Model file for the job. Use its own axes, mm. Face numbers are marked on the shaded views. A direction names the side the tool comes from. Coordinates: 2 decimals unless noted, no trailing zeros. Loops run counter-clockwise (first coordinate to the right, second up) from the corner with the lowest first, then second, coordinate; pieces in that order, holes last. Notation, with made-up numbers: (60, 71.25) -> (113, 71.25) arc R8 cw to (113, 78.25) -> close; hole circle Ø4 at (-20.75, 6). An arc over 180 degrees is marked (long way). Use one line per item in the form item = value.
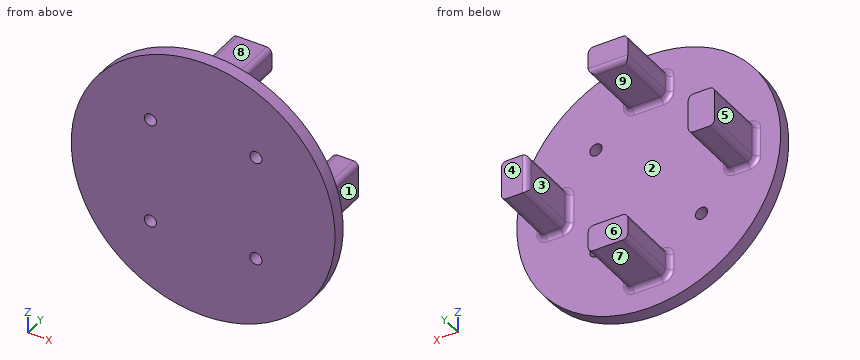
```python
from build123d import *

# Parameters (mm, degrees)
SKETCH2_R           = 63.5
SKETCH2_R_2         = 2.921
BOSS_EXTRUDE2_DEPTH = 6.35
SKETCH3_W           = 19.05
SKETCH3_H           = 12.7
SKETCH3_W_2         = 12.7
SKETCH3_H_2         = 19.05
BOSS_EXTRUDE3_DEPTH = 31.75
FILLET1_R           = 2.54


with BuildPart() as part:
    # Sketch2 → Boss-Extrude2 (new body)
    with BuildSketch(Plane(origin=(0, 0, 0), x_dir=(1, 0, 0), z_dir=(0, 1, 0))):
        with Locations(Location((0, 0, 0), (0, 0, 270))):
            Circle(SKETCH2_R)
        with Locations(Location((-25.4, 25.4, 0), (0, 0, 270))):
            Circle(SKETCH2_R_2, mode=Mode.SUBTRACT)
        with Locations(Location((25.4, 25.4, 0), (0, 0, 270))):
            Circle(SKETCH2_R_2, mode=Mode.SUBTRACT)
        with Locations(Location((25.4, -25.4, 0), (0, 0, 270))):
            Circle(SKETCH2_R_2, mode=Mode.SUBTRACT)
        with Locations(Location((-25.4, -25.4, 0), (0, 0, 270))):
            Circle(SKETCH2_R_2, mode=Mode.SUBTRACT)
    extrude(amount=BOSS_EXTRUDE2_DEPTH)

    # Sketch3 → Boss-Extrude3 (add)
    with BuildSketch(Plane(origin=(0, 6.35, 0), x_dir=(1, 0, 0), z_dir=(0, 1, 0))):
        with Locations((0, 44.831)):
            Rectangle(SKETCH3_W, SKETCH3_H)
        with Locations((0, -44.831)):
            Rectangle(SKETCH3_W, SKETCH3_H)
        with Locations((-44.971451378, 0)):
            Rectangle(SKETCH3_W_2, SKETCH3_H_2)
        with Locations((44.971451378, 0)):
            Rectangle(SKETCH3_W_2, SKETCH3_H_2)
    extrude(amount=BOSS_EXTRUDE3_DEPTH)

    # Fillet1
    fillet1_edges = [part.edges().sort_by_distance(p)[0] for p in [
        (9.525, 6.35, -44.831),
        (9.525, 22.225, -38.481),
        (0, 6.35, -51.181),
        (9.525, 22.225, -51.181),
        (-9.525, 6.35, -44.831),
        (-9.525, 22.225, -51.181),
        (0, 6.35, -38.481),
        (-9.525, 22.225, -38.481),
        (-9.525, 6.35, 44.831),
        (-9.525, 22.225, 38.481),
        (0, 6.35, 51.181),
        (-9.525, 22.225, 51.181),
        (9.525, 6.35, 44.831),
        (9.525, 22.225, 51.181),
        (0, 6.35, 38.481),
        (9.525, 22.225, 38.481),
        (0, 38.1, 38.481),
        (-38.621451378, 6.35, 0),
        (-38.621451378, 22.225, 9.525),
        (-44.971451378, 6.35, -9.525),
        (-38.621451378, 22.225, -9.525),
        (-51.321451378, 6.35, 0),
        (-51.321451378, 22.225, -9.525),
        (-44.971451378, 6.35, 9.525),
        (-51.321451378, 22.225, 9.525),
        (44.971451378, 6.35, -9.525),
        (51.321451378, 22.225, -9.525),
        (38.621451378, 6.35, 0),
        (38.621451378, 22.225, -9.525),
        (44.971451378, 6.35, 9.525),
        (38.621451378, 22.225, 9.525),
        (51.321451378, 6.35, 0),
        (51.321451378, 22.225, 9.525),
        (38.621451378, 38.1, 0),
    ]]
    fillet(fillet1_edges, radius=FILLET1_R)


solid = part.part
```
Q1. Wall check: line 1 along Z through (x, y) = (-0.5, 22); line 2 along X through (y, z) = (3.75, 25.4); line 3 along X through (y, z) = (29.5, -46) (3 decimals). Give the ranges that are in metal, low to high.
Result:
line_1 = -51.18 to -38.48, 38.48 to 51.18
line_2 = -58.2 to -28.32, -22.48 to 22.48, 28.32 to 58.2
line_3 = -9.525 to 9.525
Q2. Pin check, flat tips, straight feed: pin 1 Ø4 at (y, z) = (19.5, 0.5) entering from +X; pin 2 Ø5 at (x, y) = (2.5, 33.5) entering from +Z; pin 3 Ø6.5 at (x, z) = (-25.4, -25.4) entering from -Y; pin 4 Ø4 at (x, y) = (46, 30.5) entering from -Z (3 decimals). Stop position of each tip, or through.
Result:
pin_1 = 51.32
pin_2 = 51.18
pin_3 = 0
pin_4 = -9.525
Q3. Band-saw the part on D-D, the plane z = 0. Write the cut outline in (x, y).
Result:
outline = (-63.5, 0) -> (63.5, 0) -> (63.5, 6.35) -> (53.86, 6.35) arc R2.54 cw to (51.32, 8.89) -> (51.32, 38.1) -> (41.16, 38.1) arc R2.54 ccw to (38.62, 35.56) -> (38.62, 8.89) arc R2.54 cw to (36.08, 6.35) -> (-36.08, 6.35) arc R2.54 cw to (-38.62, 8.89) -> (-38.62, 38.1) -> (-51.32, 38.1) -> (-51.32, 8.89) arc R2.54 cw to (-53.86, 6.35) -> (-63.5, 6.35) -> close
Q4. Band-saw the part on A-A, the plane y = 20. State how many separate pieces and enclosed holes the cut face has, and give its area (3 significant figures).
Result:
separate_pieces = 4
enclosed_holes = 0
area = 946 mm2
Q5. Mould opens along Z. For the marked faces 6, 7, 8 and 9 say: released by +Z, released by -Z, zero draft, split by the parting line, or undercut.
Result:
face_6 = zero draft
face_7 = released by -Z
face_8 = released by +Z
face_9 = undercut
Q6. Band-saw the part on C-C, the plane x = 0. Write the cut outline in (y, z).
Result:
outline = (0, -63.5) -> (6.35, -63.5) -> (6.35, -53.72) arc R2.54 cw to (8.89, -51.18) -> (38.1, -51.18) -> (38.1, -38.48) -> (8.89, -38.48) arc R2.54 cw to (6.35, -35.94) -> (6.35, 35.94) arc R2.54 cw to (8.89, 38.48) -> (35.56, 38.48) arc R2.54 ccw to (38.1, 41.02) -> (38.1, 51.18) -> (8.89, 51.18) arc R2.54 cw to (6.35, 53.72) -> (6.35, 63.5) -> (0, 63.5) -> close
Q7. Which spindle directions (+Z, -Z, +X, -X, +Y, -Y) get a long thin tool onto all of the face, cutting with end or side? Do the marked faces 1, 2, 3, 4 and 5. Say none if no direction does.
Result:
face_1 = +Z, -Z, +X, +Y
face_2 = +Y
face_3 = +Z, -Z, +Y
face_4 = +Z, -Z, +X, -X, +Y
face_5 = +Z, -Z, -X, +Y
Q8. Band-saw the part on B-B, the plane x = -25.4. Write the cut outline in (y, z).
Result:
outline = (0, -58.2) -> (6.35, -58.2) -> (6.35, -28.32) -> (0, -28.32) -> close; (0, -22.48) -> (6.35, -22.48) -> (6.35, 22.48) -> (0, 22.48) -> close; (0, 28.32) -> (6.35, 28.32) -> (6.35, 58.2) -> (0, 58.2) -> close
